```python
from build123d import *

# Parameters (mm, degrees)
SKETCH1_R           = 10
BOSS_EXTRUDE1_DEPTH = 8
SKETCH2_R           = 2.65
CUT_EXTRUDE1_DEPTH  = 8
SKETCH3_R           = 5
CUT_EXTRUDE2_DEPTH  = 5
CUT_EXTRUDE2_TAPER  = 26


with BuildPart() as part:
    # Sketch1 → Boss-Extrude1 (new body)
    with BuildSketch(Plane.XY):
        Circle(SKETCH1_R)
    extrude(amount=BOSS_EXTRUDE1_DEPTH)

    # Sketch2 → Cut-Extrude1 (cut)
    with BuildSketch(Plane(origin=(0, 0, 0), x_dir=(-1, 0, 0), z_dir=(0, 0, -1))):
        Circle(SKETCH2_R)
    extrude(amount=-CUT_EXTRUDE1_DEPTH, mode=Mode.SUBTRACT)

    # Sketch3 → Cut-Extrude2 (cut)
    with BuildSketch(Plane(origin=(0, 0, 0), x_dir=(-1, 0, 0), z_dir=(0, 0, -1))):
        Circle(SKETCH3_R)
    extrude(amount=-CUT_EXTRUDE2_DEPTH, taper=CUT_EXTRUDE2_TAPER, mode=Mode.SUBTRACT)


solid = part.part
```
Check sheet for the modelled part. Datum: model origin and axes. Units: mm. Round coordinates to 2 decimals unless told otherwise and drop trailing zeros. Order: outer loops, then holes, each group sorted by start corner. A loop starts at its lowest first (then second) coordinate and runs counter-clockwise, first axis right, second up.
1) Go/stop test with flat-tipped pins: pin 1 Ø8 at (x, y) = (0.5, 4) entering from -Z; pin 2 Ø1 at (y, z) = (6, 2) entering from +X. Record where each tip stops, or that it passes through.
2) Section check B-B (z = 6). Record the boundary of the cut face in (x, y).
3) Section check C-C (y = -5.5). Record the boundary of the cut face in (x, z), and give its area (3 significant figures).
4) Scan lines: line 1 (Y direction, x = 0, z = 6.65); line 2 (X direction, y = -1.25, z = 5.75); line 3 (Y direction, x = 2.25, z = 4.25). Record each from-to range of solid material in increasing order.
5) Section check A-A (x = 0). Record the boundary of the cut face in (y, z), and give its area (3 significant figures).
6) Mould release check, pull along Y, two halves, no side actions. Record for faces 1 (the conical face through (2.4, -1.84, 4.05)), 2 (the flat face through (2, -2, 8)), 3 (the cylindrical face through (-2.17, -9.76, 3.94)): +Y half, -Y half, draft (parallel to the pull), parting line (faces both ways), or undercut.
7) Section check D-D (x = 8.5). Record the boundary of the cut face in (y, z).
Result:
1. pin 1: stops at z = 0
1. pin 2: stops at x = 8.35
2. outline: circle Ø20 at (0, 0); hole circle Ø5.3 at (0, 0)
3. outline: (-8.35, 0) - (8.35, 0) - (8.35, 8) - (-8.35, 8) - close
3. area: 134 mm2
4. line 1: y = -10 to -2.65, 2.65 to 10
4. line 2: x = -9.92 to -2.34, 2.34 to 9.92
4. line 3: y = -9.74 to -1.87, 1.87 to 9.74
5. outline: (-10, 0) - (-5, 0) - (-2.65, 4.82) - (-2.65, 8) - (-10, 8) - close; (2.65, 4.82) - (5, 0) - (10, 0) - (10, 8) - (2.65, 8) - close
5. area: 106 mm2
6. face 1: undercut
6. face 2: draft
6. face 3: parting line
7. outline: (-5.27, 0) - (5.27, 0) - (5.27, 8) - (-5.27, 8) - close
